Part print with two shaded views. Sizes in mm from the minimum x, y, z corner. A direction names the side the tool comes from. Round coordinates to 2 decimals unless told otherwise and drop trailing zeros. Write each loop counter-clockwise with the first axis right and the second up, starting at its lowest first coordinate (ties: lowest second). Pieces come first, ordered by that corner, then holes. Notation, with made-up numbers: M 43.25,-3 L 71.25,-3 A21 ccw 71.25,13 Z; hole C 2.25,-27 d6. An arc over 180 degrees is marked long. One line per question, with ' | ' between items. Start each with the question number.
1) Saw through at D-D (x = 49.5). List the corners of the cut face in (y, z), plus the area to 3 significant figures.
2) Saw through at A-A (z = 42). List the corners of the cut face in (x, y) (1 decimal).
3) Saw through at B-B (y = 8). List the corners of the cut face in (x, z).
4) Wall check: probe 1 along Y at (x, z) = (39.5, 27.5); probe 2 along Y at (x, z) = (38, 17.5); probe 3 along Y at (x, z) = (24.5, 43). Give the ranges that are in metal, low to high. Write a range as [from, to].
5) Mould opens along Y. For the marked faces 4, 5 and 6 say: pulls with the +Y half, pulls with the -Y half, needs draft (parallel to the pull), parting line crosses it, or undercut.
6) Saw through at C-C (x = 44). List the corners of the cut face in (y, z) (1 decimal), plus the area to 3 significant figures.
7) Drop a flat-ended pin along its axis: pin 1 Ø12 at (y, z) = (24, 34) entering from +X. Give the stop position or say it passes through.
8) Tool access for the marked faces 1, 2 and 3: list every direction of +Z, -Z, +X, -X, +Y, -Y with a clear straight run to the whole face (end or side of a thin tool).
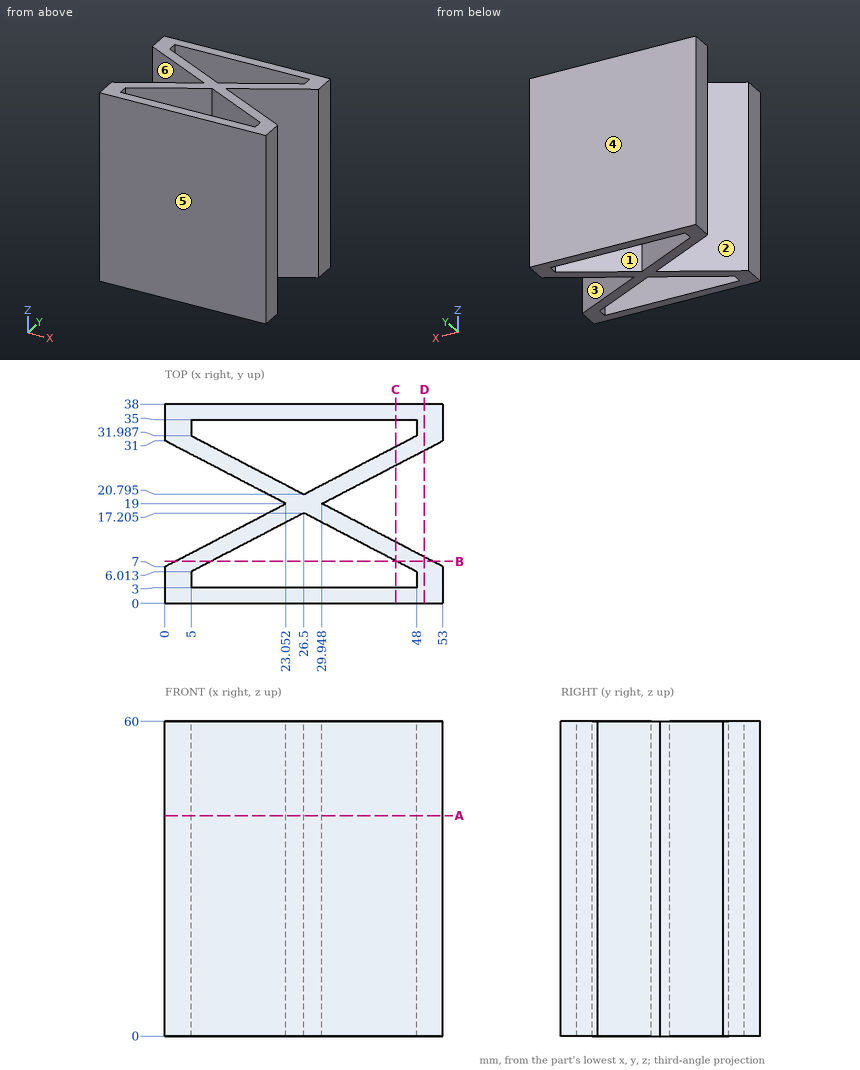
Answer key:
1) outline: M 0,0 L 8.82,0 L 8.82,60 L 0,60 Z; M 29.18,0 L 38,0 L 38,60 L 29.18,60 Z | area: 1,060 mm2
2) outline: M 0,0 L 53,0 L 53,7 L 29.9,19 L 53,31 L 53,38 L 0,38 L 0,31 L 23.1,19 L 0,7 Z; hole M 5,3 L 48,3 L 48,6 L 26.5,17.2 L 5,6 Z; hole M 5,32 L 26.5,20.8 L 48,32 L 48,35 L 5,35 Z
3) outline: M 1.92,0 L 8.82,0 L 8.82,60 L 1.92,60 Z; M 44.18,0 L 51.08,0 L 51.08,60 L 44.18,60 Z
4) probe 1: y = [0, 3], [10.44, 14.03], [23.97, 27.56], [35, 38] | probe 2: y = [0, 3], [11.22, 14.81], [23.19, 26.78], [35, 38] | probe 3: y = [0, 3], [16.16, 21.84], [35, 38]
5) face 4: pulls with the +Y half | face 5: pulls with the -Y half | face 6: undercut
6) outline: M 0,0 L 3,0 L 3,60 L 0,60 Z; M 8.1,0 L 11.7,0 L 11.7,60 L 8.1,60 Z; M 26.3,0 L 29.9,0 L 29.9,60 L 26.3,60 Z; M 35,0 L 38,0 L 38,60 L 35,60 Z | area: 791 mm2
7) pin 1: stops at x = 51.08
8) face 1: +Z, -Z | face 2: +Z, -Z, -X | face 3: +Z, -Z, +X
